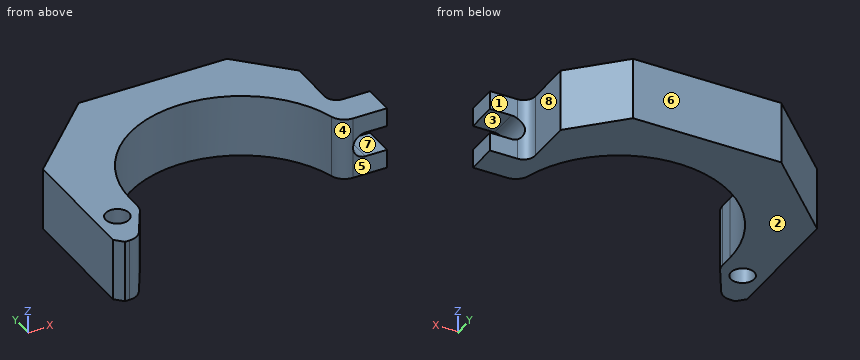
```python
from build123d import *

# Parameters (mm, degrees)
SKETCH_1_R          = 3
EXTRUDE_1_DEPTH     = 16
CHAMFER_1_SIZE      = 6
CHAMFER_1_SIZE2     = 10.392304845
SKETCH_2_W          = 70.200678886
SKETCH_2_H          = 11.369261619
CUT_EXTRUDE_1_DEPTH = 56.506756346
CHAMFER_2_SIZE      = 20
SKETCH_4_W          = 15.06489792
SKETCH_4_H          = 29.640391265
CUT_EXTRUDE_2_DEPTH = 56.506756346
CHAMFER_3_SIZE      = 12
FILLET_1_R          = 3
FILLET_2_R          = 4
FILLET_3_R          = 4
FILLET_4_R          = 4
CHAMFER_4_SIZE      = 2
CUT_EXTRUDE_3_DEPTH = 10


with BuildPart() as part:
    # 草图1 → 凸台-拉伸1 (new body)
    with BuildSketch(Plane.XY):
        with BuildLine():
            Line((-40, 20), (40, 20))
            Line((40, 20), (40, -20))
            Line((40, -20), (28.5, -20))
            ThreePointArc((28.5, -20), (0, 8.5), (-28.5, -20))
            Line((-28.5, -20), (-28.5, -35))
            Line((-28.5, -35), (-40, -35))
            Line((-40, -35), (-40, -20))
            Line((-40, -20), (-40, 20))
        make_face()
        with Locations((-34.5, -25)):
            Circle(SKETCH_1_R, mode=Mode.SUBTRACT)
    extrude(amount=EXTRUDE_1_DEPTH)

    # 倒角1
    chamfer_1_edges = [part.edges().sort_by_distance(p)[0] for p in [
        (-28.5, -35, 8),
    ]]
    chamfer_1_side = [part.faces().sort_by_distance(p)[0] for p in [
        (-34.25, -35, 8),
    ]]
    chamfer(chamfer_1_edges, length=CHAMFER_1_SIZE, length2=CHAMFER_1_SIZE2, reference=chamfer_1_side[0])

    # 草图2 → 切除-拉伸1 (cut, through all)
    with BuildSketch(Plane.XY.offset(16)):
        with Locations((17.588251777, -20.68463081)):
            Rectangle(SKETCH_2_W, SKETCH_2_H)
    extrude(amount=-CUT_EXTRUDE_1_DEPTH, mode=Mode.SUBTRACT)

    # 倒角2
    chamfer_2_edges = [part.edges().sort_by_distance(p)[0] for p in [
        (-40, 20, 8),
    ]]
    chamfer(chamfer_2_edges, length=CHAMFER_2_SIZE)

    # 草图4 → 切除-拉伸2 (cut, through all)
    with BuildSketch(Plane.XY.offset(16)):
        with Locations((37.53244896, 7.820195633)):
            Rectangle(SKETCH_4_W, SKETCH_4_H)
    extrude(amount=-CUT_EXTRUDE_2_DEPTH, mode=Mode.SUBTRACT)

    # 倒角3
    chamfer_3_edges = [part.edges().sort_by_distance(p)[0] for p in [
        (30, 20, 8),
    ]]
    chamfer(chamfer_3_edges, length=CHAMFER_3_SIZE)

    # 圆角1
    fillet_1_edges = [part.edges().sort_by_distance(p)[0] for p in [
        (30, -7, 8),
    ]]
    fillet(fillet_1_edges, radius=FILLET_1_R)

    # 圆角2
    fillet_2_edges = [part.edges().sort_by_distance(p)[0] for p in [
        (-28.5, -24.607695155, 8),
    ]]
    fillet(fillet_2_edges, radius=FILLET_2_R)

    # 圆角3
    fillet_3_edges = [part.edges().sort_by_distance(p)[0] for p in [
        (-34.5, -35, 8),
    ]]
    fillet(fillet_3_edges, radius=FILLET_3_R)

    # 圆角4
    fillet_4_edges = [part.edges().sort_by_distance(p)[0] for p in [
        (28.057975693, -15, 8),
    ]]
    fillet(fillet_4_edges, radius=FILLET_4_R)

    # 倒角4
    chamfer_4_edges = [part.edges().sort_by_distance(p)[0] for p in [
        (-40, -35, 8),
    ]]
    chamfer(chamfer_4_edges, length=CHAMFER_4_SIZE)

    # 草图5 → 切除-拉伸3 (cut)
    with BuildSketch(Plane.XZ.offset(15)):
        with BuildLine():
            Line((34.5, 11.2), (41.178159838, 11.2))
            ThreePointArc((41.178159838, 11.2), (44.378159838, 8), (41.178159838, 4.8))
            Line((41.178159838, 4.8), (34.5, 4.8))
            ThreePointArc((34.5, 4.8), (31.3, 8), (34.5, 11.2))
        make_face()
    extrude(amount=-CUT_EXTRUDE_3_DEPTH, mode=Mode.SUBTRACT)


solid = part.part
```
Design review of the part built by this model. Coordinates are the model's own, in mm. Face numbers are marked on the shaded views. A direction names the side the tool comes from. Give positions to 0.01 mm unless a question says otherwise; leave off trailing zeros. Order: outer loops, then holes, each group sorted by start corner. A loop starts at its lowest first (then second) coordinate and runs counter-clockwise, first axis right, second up. Notation, with made-up numbers: M 21,31 L 74,31 A16 ccw 74,59 Z; hole C 70,64.5 d11. An arc over 180 degrees is marked long. One line per question, with ' | ' between items. Start each with the question number.
Q1. The part is to be moulded in two halves that separate along Z. For the marked faces 1, 2 and 3, say which applies: +Z half, -Z half, draft (parallel to the pull), parting line (faces both ways), or undercut.
Q2. We need section C-C (y = 12). Write out the cut boundary in (x, z).
Q3. For L1, parallel to Y at x = -34.5, z = 9; L2, parallel to X at y = 4, z = 13.5; L3, parallel to X at y = -11, z = 1.5, list the stretches that pass through material, from the lowest coordinate up. Write a range as [from, to].
Q4. Machinability: for the marked faces 4, 5, 6, 7 and 8, which of the approach directions +Z, -Z, +X, -X, +Y, -Y give a long, thin tool a straight path to every point of the face, cutting with its end or side? Answer none if there is none.
Q5. We need section A-A (z = 4). Write out the cut boundary in (x, y), plus the area to 3 significant figures.
Q6. For pin 1 Ø4 at (x, z) = (-8, 11) entering from -Y; pin 2 Ø1.6 at (x, z) = (38, 13.5) entering from +Y; pin 3 Ø2 at (x, z) = (12.5, 12.5) entering from -Y, all flat-tipped, find the tip position at first contact; note any pin that passes through.
Q7. We need section D-D (z = 8). Write out the cut boundary in (x, y).
Q8. We need section B-B (y = -5). Write out the cut boundary in (x, z).
Returned:
1) face 1: draft | face 2: -Z half | face 3: undercut
2) outline: M -28,0 L 26,0 L 26,16 L -28,16 Z
3) L1: [-34.27, -28], [-22, 5.5] | L2: [-36, -15.37], [15.37, 30] | L3: [-40, -27.04], [27.04, 40]
4) face 4: +Z, -Z, -Y | face 5: +Z, -Z, +X, -Y | face 6: +Z, -Z, +X, -X, +Y | face 7: +X, +Y, -Y | face 8: +Z, -Z, +X, +Y
5) outline: M -40,-33 L -38,-35 L -36.81,-35 A4 ccw -33.35,-33 L -29.04,-25.54 A4 ccw -28.5,-23.54 L -28.5,-20 A28.5 cw 27.39,-12.11 A4 ccw 31.23,-15 L 40,-15 L 40,-7 L 33,-7 A3 cw 30,-4 L 30,8 L 18,20 L -20,20 L -40,0 Z; hole C -34.5,-25 d6 | area: 1,430 mm2
6) pin 1: y = 6.69 | pin 2: y = -7 | pin 3: y = 5.1
7) outline: M -40,-33 L -38,-35 L -36.81,-35 A4 ccw -33.35,-33 L -29.04,-25.54 A4 ccw -28.5,-23.54 L -28.5,-20 A28.5 cw 27.39,-12.11 A4 ccw 31.23,-15 L 31.3,-15 L 31.3,-6.47 A3 cw 30,-4 L 30,8 L 18,20 L -20,20 L -40,0 Z; hole C -34.5,-25 d6
8) outline: M -40,0 L -24.23,0 L -24.23,16 L -40,16 Z; M 24.23,0 L 30.17,0 L 30.17,16 L 24.23,16 Z
